Build history of the part. All positions in model axes, mm. A direction names the side the tool comes from. Round coordinates to 2 decimals unless told otherwise and drop trailing zeros. Loops run counter-clockwise (first coordinate to the right, second up) from the corner with the lowest first, then second, coordinate; pieces in that order, holes last.
from build123d import *

# Parameters (mm, degrees)
SKETCH_2_W          = 50
SKETCH_2_H          = 7.55
SKETCH_2_R          = 1.6
EXTRUDE_1_DEPTH     = 4.9
SKETCH_3_W          = 23.885574904
SKETCH_3_H          = 13.680093874
SKETCH_3_R          = 1.6
EXTRUDE_2_DEPTH     = 10
SKETCH_4_W          = 10
SKETCH_4_H          = 10.264550668
CUT_EXTRUDE_1_DEPTH = 48.143107127
SKETCH_6_W          = 14
SKETCH_6_H          = 41
SKETCH_6_R          = 1.6
EXTRUDE_4_DEPTH     = 7.5
SKETCH_7_W          = 8
SKETCH_7_H          = 41
CUT_EXTRUDE_2_DEPTH = 10
EXTRUDE_5_DEPTH     = 12.5
CHAMFER_1_SIZE      = 5


with BuildPart() as part:
    # Sketch 2 → Extrude 1 (new, symmetric)
    with BuildSketch(Plane(origin=(0, 0, 0), x_dir=(0, 0, -1), z_dir=(1, 0, 0))):
        with Locations((19.75, 0)):
            Rectangle(SKETCH_2_W, SKETCH_2_H)
        Circle(SKETCH_2_R, mode=Mode.SUBTRACT)
        with Locations((7, 0)):
            Circle(SKETCH_2_R, mode=Mode.SUBTRACT)
        with Locations((32.5, 0)):
            Circle(SKETCH_2_R, mode=Mode.SUBTRACT)
        with Locations((39.5, 0)):
            Circle(SKETCH_2_R, mode=Mode.SUBTRACT)
    extrude(amount=EXTRUDE_1_DEPTH, both=True)

    # Sketch 3 → Extrude 2 (add, symmetric)
    with BuildSketch(Plane(origin=(0, 0, 0), x_dir=(0, 0, -1), z_dir=(1, 0, 0))):
        with Locations((14.057212548, 10.615046937)):
            Rectangle(SKETCH_3_W, SKETCH_3_H)
        with Locations((7, 13)):
            Circle(SKETCH_3_R, mode=Mode.SUBTRACT)
        with Locations((20, 13)):
            Circle(SKETCH_3_R, mode=Mode.SUBTRACT)
    extrude(amount=EXTRUDE_2_DEPTH, both=True)

    # Sketch 4 → Cut-Extrude 1 (cut, through all)
    with BuildSketch(Plane.XY.offset(-2.114425096)):
        with Locations((0, 12.32281854)):
            Rectangle(SKETCH_4_W, SKETCH_4_H)
    extrude(amount=-CUT_EXTRUDE_1_DEPTH, mode=Mode.SUBTRACT)



with BuildPart() as body_2:
    # Sketch 6 → Extrude 4 (new, symmetric)
    with BuildSketch(Plane(origin=(0, 0, 0), x_dir=(0, 0, -1), z_dir=(1, 0, 0))):
        with Locations((67, -0.9)):
            Rectangle(SKETCH_6_W, SKETCH_6_H)
        with Locations((70, 3.6)):
            Circle(SKETCH_6_R, mode=Mode.SUBTRACT)
        with Locations((70, 13.6)):
            Circle(SKETCH_6_R, mode=Mode.SUBTRACT)
        with Locations((70, -6.4)):
            Circle(SKETCH_6_R, mode=Mode.SUBTRACT)
    extrude(amount=EXTRUDE_4_DEPTH, both=True)

    # Sketch 7 → Cut-Extrude 2 (cut)
    with BuildSketch(Plane.XY.offset(-74)):
        with Locations((0, -0.9)):
            Rectangle(SKETCH_7_W, SKETCH_7_H)
    extrude(amount=CUT_EXTRUDE_2_DEPTH, mode=Mode.SUBTRACT)


with BuildPart() as part_1:
    add(part.part)

    add(body_2.part)  # Extrude 5 merges body 2
    # Sketch 8 → Extrude 5 (add, symmetric)
    with BuildSketch(Plane(origin=(0, 0, 0), x_dir=(0, 0, -1), z_dir=(1, 0, 0))):
        Polygon((44.75, -3.775), (44.75, -9.506092627), (60, -9.506092627), (60, -17.854611286), (18.724521107, -17.854611286), (18.724521107, -3.775), align=None)
    extrude(amount=EXTRUDE_5_DEPTH, both=True)

    # Chamfer 1
    chamfer_1_edges = [part_1.edges().sort_by_distance(p)[0] for p in [
        (-7.5, -13.680351956, -60),
        (7.5, -13.680351956, -60),
    ]]
    chamfer(chamfer_1_edges, length=CHAMFER_1_SIZE - 0.0001)  # a hair under: the kernel refuses the full size


solid = part_1.part
(1) Slice it at C-C on x = 6. List the corners of the cut face in (y, z) (3 decimals).
Responses:
outline: (-21.4, -74) - (19.6, -74) - (19.6, -60) - (-9.506, -60) - (-9.506, -44.75) - (-3.775, -44.75) - (-3.775, -18.725) - (-17.855, -18.725) - (-17.855, -60) - (-21.4, -60) - close; (3.775, -26) - (17.455, -26) - (17.455, -2.114) - (3.775, -2.114) - close; hole circle Ø3.2 at (-6.4, -70); hole circle Ø3.2 at (3.6, -70); hole circle Ø3.2 at (13, -20); hole circle Ø3.2 at (13, -7); hole circle Ø3.2 at (13.6, -70)
(2) Probe line 1 (Y direction, x = -6.5, z = -70); line 2 (Y direction, x = 8.95, z = -20) (3 decimals); line 3 (Z direction, x = 6.25, y = 15.5). List the from-to ranges inside material, lowest first.
Responses:
line 1: y = -21.4 to -8, -4.8 to 2, 5.2 to 12, 15.2 to 19.6
line 2: y = -17.855 to -3.775, 3.775 to 11.4, 14.6 to 17.455
line 3: z = -74 to -60, -26 to -2.11
(3) Pull direction X, two halves, no side cores. Call faces 1 (the face through (4, -1, -69)), 2 (the face through (7.5, -1, -67)), 3 (the face through (5.726, 14.081, -71.526)): +X half, -X half, draft (parallel to the pull), parting line (faces both ways), or undercut.
Responses:
face 1: undercut
face 2: +X half
face 3: draft
(4) Which spindle directions (+Z, -Z, +X, -X, +Y, -Y) get a long thin tool onto all of the face, cutting with end or side? Do faces 4 (the face through (0, -11, -18.725)), 5 (the face through (-4, -1, -69)), 6 (the face through (0, 3.775, -35)), 7 (the face through (-10, 11, -14)), 8 (the face through (7, 3.775, -14)). Say none if no direction does.
Responses:
face 4: +Z, +X, -X, -Y
face 5: -Z, +Y, -Y
face 6: +X, -X, +Y
face 7: +Z, -Z, -X, +Y
face 8: +Z, +X
(5) Slice it at D-D on z = -7. List the corners of the cut face in (x, y) (3 decimals), plus the area to 3 significant figures.
Responses:
outline: (-10, 3.775) - (-4.9, 3.775) - (-4.9, 1.6) - (4.9, 1.6) - (4.9, 3.775) - (10, 3.775) - (10, 11.4) - (5, 11.4) - (5, 7.191) - (-5, 7.191) - (-5, 11.4) - (-10, 11.4) - close; (-10, 14.6) - (-5, 14.6) - (-5, 17.455) - (-10, 17.455) - close; (-4.9, -3.775) - (4.9, -3.775) - (4.9, -1.6) - (-4.9, -1.6) - close; (5, 14.6) - (10, 14.6) - (10, 17.455) - (5, 17.455) - close
area: 182 mm2
(6) Pin check, flat tips, straight feed: P1, Ø12, axis at x = 6.5, z = -7.5, coming from the -Y side (3 decimals); P2, Ø11, axis at y = 8.5, z = -11, coming from the -X side; P3, Ø2.5, axis at y = 0.5, z = -20, coming from the -X side; P4, Ø3, axis at y = 3.6, z = -70, coming from the +X side. Stop position of each tip, or through.
Responses:
P1: stops at y = -3.775
P2: stops at x = -10
P3: stops at x = -4.9
P4: passes through
(7) Slice it at A-A on y = -6.4. List the corners of the cut face in (x, z), plus the area to 3 significant figures.
Responses:
outline: (-12.5, -44.75) - (12.5, -44.75) - (12.5, -18.72) - (-12.5, -18.72) - close; (-7.5, -74) - (-4, -74) - (-4, -71.6) - (-7.5, -71.6) - close; (-7.5, -68.4) - (-4, -68.4) - (-4, -64) - (4, -64) - (4, -68.4) - (7.5, -68.4) - (7.5, -60) - (-7.5, -60) - close; (4, -74) - (7.5, -74) - (7.5, -71.6) - (4, -71.6) - close
area: 758 mm2
(8) Slice it at B-B on z = -70. Count the separate pieces of the cut face and the enclosed holes in it, plus the area to 3 significant figures.
Responses:
separate pieces: 8
enclosed holes: 0
area: 220 mm2
